Here's how the part is built. I have some questions about the finished solid (model axes, mm). Coordinates: 2 decimals unless noted, no trailing zeros. Write each loop counter-clockwise with the first axis right and the second up, starting at its lowest first coordinate (ties: lowest second). Pieces come first, ordered by that corner, then holes.
(1) For pin 1 Ø2 at (y, z) = (3, 130.5) entering from -X; pin 2 Ø1 at (x, z) = (-1.5, -176) entering from -Y; pin 3 Ø2 at (y, z) = (-4, 129) entering from +X, each with a flat end and sliding along its axis, tell me the tip position at first contact or that it passes through.
(2) Please list where these lines run through material, in increasing order: probe 1 along Y at (x, z) = (-0.75, -168.5); probe 2 along X at (y, z) = (-0.5, -220.5); probe 3 along Z at (x, y) = (-2, -1.5).
(3) Imagine slicing it at B-B, the plane x = -3. List the corners of the cut face in (y, z) for me.
(4) Imagine slicing it at A-A, the plane z = -235. List the corners of the cut face in (x, y) for me.
```python
from build123d import *

# Parameters (mm, degrees)
SKETCH3_R           = 5
BOSS_EXTRUDE1_DEPTH = 300
REVOLVE3_ANGLE      = 180


with BuildPart() as part:
    # Sketch3 → Boss-Extrude1 (new body)
    with BuildSketch(Plane.XY):
        Circle(SKETCH3_R)
    boss_extrude1 = extrude(amount=BOSS_EXTRUDE1_DEPTH)

    # Sketch4 → Revolve3 (revolve)
    with BuildSketch(Plane.XY.offset(300)):
        with BuildLine():
            Line((0, 5), (0, -5))
            ThreePointArc((0, -5), (-5, 0), (0, 5))
        make_face()
    revolve3 = revolve(axis=Axis((0, 5, 300), (0, 1, 0)), revolution_arc=REVOLVE3_ANGLE)

    # Mirror2: Boss-Extrude1, Revolve3 across plane
    add(boss_extrude1.mirror(Plane.XY))
    add(revolve3.mirror(Plane.XY))


solid = part.part
```
Recorded:
1. pin 1: stops at x = -4.58
1. pin 2: stops at y = -4.9
1. pin 3: stops at x = 4
2. probe 1: y = -4.94 to 4.94
2. probe 2: x = -4.97 to 4.97
2. probe 3: z = -304.33 to 304.33
3. outline: (-4, -300) arc R4 ccw to (4, -300) - (4, 300) arc R4 ccw to (-4, 300) - close
4. outline: circle Ø10 at (0, 0)
